```python
from build123d import *

# Parameters (mm, degrees)
BOSS_EXTRUDE1_DEPTH = 1.5


with BuildPart() as part:
    # Sketch1 → Boss-Extrude1 (new, symmetric)
    with BuildSketch(Plane(origin=(0, 0, 0), x_dir=(0, 0, -1), z_dir=(1, 0, 0))):
        with BuildLine():
            Line((0, 0), (-5, 0))
            Line((-5, 0), (-5, -3))
            Line((-5, -3), (-15, -3))
            Line((-15, -3), (-15, 0))
            Line((-15, 0), (-25, 0))
            Line((-25, 0), (-25, -3))
            Line((-25, -3), (-35, -3))
            Line((-35, -3), (-35, 0))
            Line((-35, 0), (-40, 0))
            Line((-40, 0), (-40, 5))
            ThreePointArc((-40, 5), (-29.748737342, 29.748737342), (-5, 40))
            Line((-5, 40), (0, 40))
            Line((0, 40), (0, 35))
            Line((0, 35), (3, 35))
            Line((3, 35), (3, 25))
            Line((3, 25), (0, 25))
            Line((0, 25), (0, 15))
            Line((0, 15), (3, 15))
            Line((3, 15), (3, 5))
            Line((3, 5), (0, 5))
            Line((0, 5), (0, 0))
        make_face()
        with BuildLine():
            Line((-8.476149614, 19.24016953), (-11.723744879, 24.86516953))
            ThreePointArc((-11.723744879, 24.86516953), (-12.867574265, 26.008998916), (-14.430074265, 26.42766953))
            Line((-14.430074265, 26.42766953), (-20.925264794, 26.42766953))
            ThreePointArc((-20.925264794, 26.42766953), (-22.487764794, 26.008998916), (-23.631594181, 24.86516953))
            Line((-23.631594181, 24.86516953), (-26.879189445, 19.24016953))
            ThreePointArc((-26.879189445, 19.24016953), (-27.297860058, 17.67766953), (-26.879189445, 16.11516953))
            Line((-26.879189445, 16.11516953), (-23.631594181, 10.49016953))
            ThreePointArc((-23.631594181, 10.49016953), (-22.487764794, 9.346340143), (-20.925264794, 8.92766953))
            Line((-20.925264794, 8.92766953), (-14.430074265, 8.92766953))
            ThreePointArc((-14.430074265, 8.92766953), (-12.867574265, 9.346340143), (-11.723744879, 10.49016953))
            Line((-11.723744879, 10.49016953), (-8.476149614, 16.11516953))
            ThreePointArc((-8.476149614, 16.11516953), (-8.057479001, 17.67766953), (-8.476149614, 19.24016953))
        make_face(mode=Mode.SUBTRACT)
    extrude(amount=BOSS_EXTRUDE1_DEPTH, both=True)


solid = part.part
```
Model file for the job. Use its own axes, mm. A direction names the side the tool comes from. Coordinates: 2 decimals unless noted, no trailing zeros. Loops run counter-clockwise (first coordinate to the right, second up) from the corner with the lowest first, then second, coordinate; pieces in that order, holes last. Notation, with made-up numbers: (58.25, 28) - (65.25, 28) arc R16 cw to (65.25, 51) - close; hole circle Ø7 at (-31.75, -13). An arc over 180 degrees is marked (long way). Answer as a JSON object with one key per item and string values. Group by question number.
(1) Two-plate mould, pull along Y, no slides. Class faces 6 (the face through (0, 30, -3)), 7 (the face through (0, 35, -1)), 8 (the face through (0, 13.3, 10.1)): released by +Y, released by -Y, zero draft, split by the parting line, or undercut.
(2) Flat gauge pins, fed straight in: pin 1 (1.5 mm diameter, centred on x = 0, z = -1.5, fed in from -Y); pin 2 (1.5 mm diameter, centred on x = -0.5, y = -1.5, fed in from -Z); pin 3 (1.5 mm diameter, centred on x = 0, z = 3.5, fed in from -Y). Where does each tip first touch, or does it go through?
(3) Cut at C-C (y = 27.5). Give the cut face in (x, z), then the cut area to 3 significant figures.
(4) Tool access for faces 1 (the face through (0.021, 22.092, 25.233)), 2 (the face through (0, -2, 15)), 3 (the face through (0, 38, 0)), 4 (the face through (0, 5, -2)), 5 (the face through (0, 25, -2)): list every direction of +Z, -Z, +X, -X, +Y, -Y with a clear straight run to the whole face (end or side of a thin tool).
(5) Cut at A-A (y = 18). Give the cut face in (x, z).
(6) Cut at D-D (y = 32.5). Give the cut face in (x, z).
(7) Probe line 1 along Z through (x, y) = (-1.1, -0.5); line 2 along Z through (x, y) = (0.4, 3); line 3 along Z through (x, y) = (-0.9, 10). List the from-to ranges inside material, lowest first.
Geometry says:
{
 "1": {"face 6": "zero draft", "face 7": "released by +Y", "face 8": "undercut"},
 "2": {"pin 1": "stops at y = 5", "pin 2": "stops at z = 5", "pin 3": "stops at y = 0"},
 "3": {"outline": "(-1.5, -3) - (1.5, -3) - (1.5, 31.81) - (-1.5, 31.81) - close", "area": "104 mm^2"},
 "4": {"face 1": "+X, -X", "face 2": "+X, -X, -Y", "face 3": "-Z, +X, -X, +Y", "face 4": "-Z, +X, -X, -Y", "face 5": "-Z, +X, -X"},
 "5": {"outline": "(-1.5, 0) - (1.5, 0) - (1.5, 8.07) - (-1.5, 8.07) - close; (-1.5, 27.28) - (1.5, 27.28) - (1.5, 37.5) - (-1.5, 37.5) - close"},
 "6": {"outline": "(-1.5, -3) - (1.5, -3) - (1.5, 26.65) - (-1.5, 26.65) - close"},
 "7": {"line 1": "z = 5 to 15, 25 to 35", "line 2": "z = 0 to 40", "line 3": "z = -3 to 12.07, 23.28 to 39.64"}
}
